Here's how the part is built. I have some questions about the finished solid (model axes, mm). Face numbers are marked on the shaded views. A direction names the side the tool comes from. Give positions to 0.01 mm unless a question says otherwise; leave off trailing zeros. Write each loop counter-clockwise with the first axis right and the second up, starting at its lowest first coordinate (ties: lowest second). Pieces come first, ordered by that corner, then holes. Notation, with made-up numbers: (-6.5, -14) - (26.5, -14) arc R23 cw to (26.5, 17) - close; hole circle Ø11 at (13.25, 46). An arc over 180 degrees is marked (long way). Use a Markdown table: item, result.
```python
from build123d import *

# Parameters (mm, degrees)
SKETCH_1_R         = 4.5
EXTRUDE_1_DEPTH    = 9
SKETCH_2_W         = 14
SKETCH_2_H         = 5
EXTRUDE_2_DEPTH    = 3
HOLE_WIZARD_M5_1_D = 4.2
FILLET_1_R         = 1


with BuildPart() as part:
    # 草图1 → 凸台-拉伸1 (new body)
    with BuildSketch(Plane.XY):
        Circle(SKETCH_1_R)
    extrude(amount=EXTRUDE_1_DEPTH)

    # 草图2 → 凸台-拉伸2 (add)
    with BuildSketch(Plane(origin=(0, 0, 0), x_dir=(-1, 0, 0), z_dir=(0, 0, -1))):
        Rectangle(SKETCH_2_W, SKETCH_2_H)
    extrude(amount=-EXTRUDE_2_DEPTH)

    # M5 螺纹孔1 (through all)
    with Locations(Plane.XY.offset(9)):
        with Locations((0, 0)):
            Hole(HOLE_WIZARD_M5_1_D / 2)

    # 圆角1
    fillet_1_edges = [part.edges().sort_by_distance(p)[0] for p in [
        (-7, -2.5, 1.5),
        (7, 2.5, 1.5),
        (-7, 2.5, 1.5),
        (-3.741657387, -2.5, 1.5),
        (3.741657387, -2.5, 1.5),
        (7, -2.5, 1.5),
        (3.741657387, 2.5, 1.5),
        (-3.741657387, 2.5, 1.5),
    ]]
    fillet(fillet_1_edges, radius=FILLET_1_R)


solid = part.part
```
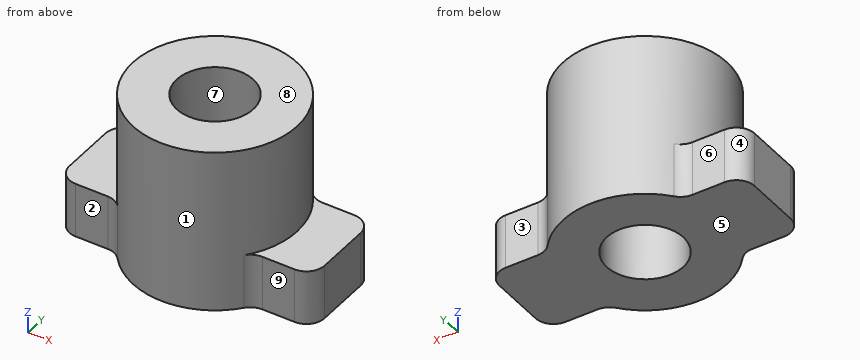
Item 1: I need wall thicknesses on line 1 along Y through (x, z) = (0, 5.5); line 2 along Z through (x, y) = (-5.25, 0.75); line 3 along X through (y, z) = (1.5, 6.25). Which ranges of each line are inside material? Lowest first, please. Write a range as [from, to].
Values:
| item | result |
|---|---|
| line 1 | y = [-4.5, -2.1], [2.1, 4.5] |
| line 2 | z = [0, 3] |
| line 3 | x = [-4.24, -1.47], [1.47, 4.24] |
Item 2: If we section it at C-C, the plane z = 2: Write out the boundary of the cut face in (x, y).
Values:
| item | result |
|---|---|
| outline | (-7, -1.5) arc R1 ccw to (-6, -2.5) - (-4.24, -2.5) arc R1 cw to (-3.47, -2.86) arc R4.5 ccw to (3.47, -2.86) arc R1 cw to (4.24, -2.5) - (6, -2.5) arc R1 ccw to (7, -1.5) - (7, 1.5) arc R1 ccw to (6, 2.5) - (4.24, 2.5) arc R1 cw to (3.47, 2.86) arc R4.5 ccw to (-3.47, 2.86) arc R1 cw to (-4.24, 2.5) - (-6, 2.5) arc R1 ccw to (-7, 1.5) - close; hole circle Ø4.2 at (0, 0) |
Item 3: If we section it at B-B, the plane y = 0: Write out the boundary of the cut face in (x, z), plus the area to 3 significant figures.
Values:
| item | result |
|---|---|
| outline | (-7, 0) - (-2.1, 0) - (-2.1, 9) - (-4.5, 9) - (-4.5, 3) - (-7, 3) - close; (2.1, 0) - (7, 0) - (7, 3) - (4.5, 3) - (4.5, 9) - (2.1, 9) - close |
| area | 58.2 mm2 |
Item 4: For the marked faces 1, 2, 3, 4 and 5, which set-ups out of +Z, -Z, +X, -X, +Y, -Y let a thin tool reach every point of the face, with its end or its side?
Values:
| item | result |
|---|---|
| face 1 | +Z |
| face 2 | +Z, -Z, -X, -Y |
| face 3 | +Z, -Z, +X, +Y |
| face 4 | +Z, -Z, -X, +Y |
| face 5 | -Z, +X, -X, +Y, -Y |
Item 5: If we section it at A-A, the plane x = 0: Write out the boundary of the cut face in (y, z).
Values:
| item | result |
|---|---|
| outline | (-4.5, 0) - (-2.1, 0) - (-2.1, 9) - (-4.5, 9) - close; (2.1, 0) - (4.5, 0) - (4.5, 9) - (2.1, 9) - close |
Item 6: Thinking about a two-plate mould opening in Y: for the marked faces 6, 7, 8 and 9, which applies, +Y half, -Y half, draft (parallel to the pull), parting line (faces both ways), or undercut?
Values:
| item | result |
|---|---|
| face 6 | +Y half |
| face 7 | undercut |
| face 8 | draft |
| face 9 | -Y half |
Item 7: Will these pins go through, and if not, where does the flat tip stop? pin 1 Ø2.5 at (x, y) = (0, 0) entering from -Z; pin 2 Ø3 at (x, y) = (-5.5, 3) entering from +Z; pin 3 Ø1.9 at (x, z) = (-5, 1.5) entering from -Y; pin 4 Ø0.5 at (x, z) = (5, 2) entering from +Y.
Values:
| item | result |
|---|---|
| pin 1 | passes through |
| pin 2 | stops at z = 3 |
| pin 3 | stops at y = -2.52 |
| pin 4 | stops at y = 2.5 |
Item 8: If we section it at D-D, the plane y = 1: Write out the boundary of the cut face in (x, z), plus the area to 3 significant figures.
Values:
| item | result |
|---|---|
| outline | (-7, 0) - (-1.85, 0) - (-1.85, 9) - (-4.39, 9) - (-4.39, 3) - (-7, 3) - close; (1.85, 0) - (7, 0) - (7, 3) - (4.39, 3) - (4.39, 9) - (1.85, 9) - close |
| area | 61.4 mm2 |
